The model under review builds one solid part; all positions refer to its coordinate system, in mm. A direction names the side the tool comes from. Coordinates: 2 decimals unless noted, no trailing zeros. Write each loop counter-clockwise with the first axis right and the second up, starting at its lowest first coordinate (ties: lowest second). Pieces come first, ordered by that corner, then holes. Notation, with made-up numbers: (61.5, 86.25) - (77.5, 86.25) arc R17 cw to (77.5, 114.25) - close; hole circle Ø4 at (-11, 1). An arc over 180 degrees is marked (long way). Put each result on its own line as item: value. Start each with the question number.
Item 1: Mouldability with a two-part tool opening along X and no side actions: class faces 5 (the face through (-14, 40, 0)), 6 (the face through (-17.8, 48.5, -15.9)), 7 (the face through (-23.846, 4.93, -7.509)) as pulls with the +X half, pulls with the -X half, needs draft (parallel to the pull), parting line crosses it, or undercut.
Item 2: Consider section A-A on x = 0. Give the boundary of the cut face in (y, z).
Item 3: For pin 1 (4.5 mm diameter, centred on x = 11.14, z = -11.14, fed in from -Y); pin 2 (3 mm diameter, centred on x = -21, z = 13.5, fed in from +Y); pin 3 (8 mm diameter, centred on y = 11.5, z = -3.5, fed in from +X), all flat-tipped, find the tip position at first contact; note any pin that passes through.
Item 4: Consider section D-D on y = 39. Give the boundary of the cut face in (x, z).
Item 5: To check wall thickness, follow L1, parallel to X at y = 2, z = 0; L2, parallel to X at y = 43, z = 13; L3, parallel to Y at x = -3, z = -21.5. State the ranges of each line that lie inside material, in increasing order. Write a range as [from, to].
Item 6: Machinability: for faces 1 (the face through (16, 10, 0)), 2 (the face through (-23, 47, -13)), 3 (the face through (11, 0, -17)), 4 (the face through (-10.31, 7.46, -13.76)), which of the approach directions +Z, -Z, +X, -X, +Y, -Y give a long, thin tool a straight path to every point of the face, cutting with its end or side? Answer none if there is none.
Item 7: Consider section B-B on y = 4. Give the boundary of the cut face in (x, z), then the cut area to 3 significant figures.
Item 8: Consider section C-C on y = 15. Give the boundary of the cut face in (x, z).
```python
from build123d import *

# Parameters (mm, degrees)
F3_D            = 3.3
F3_DEPTH        = 14.1
F3_TIP          = 0.9914200214
F2_R            = 4
F4_DEPTH        = 3
F5_R            = 2.75
F6_DEPTH        = 25
F6_COPIES_COUNT = 4
F8_R            = 2
F9_DEPTH        = 25


# Not quite as in the source:
# - a pattern or mirror of a feature is missing from the dataset's text; its kind, count and spacing are read off the source's solid


with BuildPart() as f1:
    # F0 (on Top) → F1 (revolve)
    with BuildSketch(Plane.XY):
        with BuildLine():
            Line((-25, 0), (-20, 0))
            Line((-20, 0), (-20, 5))
            Line((-20, 5), (0, 5))
            Line((0, 5), (0, 50))
            Line((0, 50), (-32, 50))
            Line((-32, 50), (-32, 40))
            Line((-32, 40), (-13, 40))
            ThreePointArc((-13, 40), (-10.8786796564, 39.1213203436), (-10, 37))
            Line((-10, 37), (-10, 13))
            ThreePointArc((-10, 13), (-10.8786796564, 10.8786796564), (-13, 10))
            Line((-13, 10), (-25, 10))
            Line((-25, 10), (-25, 0))
        make_face()
    revolve(axis=Axis((0, 27.5, 0), (0, -1, 0)))

    # F3
    with Locations(Plane(origin=(0, 50, 0), x_dir=(-1, 0, 0), z_dir=(0, 1, 0))):
        with Locations((21, -13.5), (21, 13.5), (-21, 13.5), (-21, -13.5)):
            Hole(F3_D / 2, depth=F3_DEPTH)
            with Locations((0, 0, -(F3_DEPTH + F3_TIP / 2))):  # 118° drill point
                Cone(0, F3_D / 2, F3_TIP, mode=Mode.SUBTRACT)

    # F2 (on face) → F4 (cut)
    with BuildSketch(Plane(origin=(0, 50, 0), x_dir=(-1, 0, 0), z_dir=(0, 1, 0))):
        with Locations((21, -13.5)):
            Circle(F2_R)
        with Locations((-21, 13.5)):
            Circle(F2_R)
    extrude(amount=-F4_DEPTH, mode=Mode.SUBTRACT)

    # F5 (on face) → F6 (cut)
    with BuildSketch(Plane.XZ.offset(-5)):
        with Locations((11.1369318037, -11.1369318037)):
            Circle(F5_R)
    f6 = extrude(amount=-F6_DEPTH, mode=Mode.SUBTRACT)

    # F6_copies: F6 ×4 about axis
    f6_copies_axis = Axis((0, 0, 0), (0, 1, 0))
    for i in range(1, F6_COPIES_COUNT):
        add(f6.rotate(f6_copies_axis, i * 360 / F6_COPIES_COUNT), mode=Mode.SUBTRACT)

    # F8 (on face) → F9 (cut)
    with BuildSketch(Plane.XZ.offset(-5)):
        with Locations((0, 15.75)):
            Circle(F8_R)
    extrude(amount=-F9_DEPTH, mode=Mode.SUBTRACT)


solid = f1.part
```
Report:
1. face 5: needs draft
1. face 6: undercut
1. face 7: parting line crosses it
2. outline: (0, -25) - (10, -25) - (10, -13) arc R3 cw to (13, -10) - (37, -10) arc R3 cw to (40, -13) - (40, -32) - (50, -32) - (50, 32) - (40, 32) - (40, 13) arc R3 cw to (37, 10) - (13, 10) arc R3 cw to (10, 13) - (10, 13.75) - (5, 13.75) - (5, -20) - (0, -20) - close; (0, 20) - (5, 20) - (5, 17.75) - (10, 17.75) - (10, 25) - (0, 25) - close
3. pin 1: y = 40
3. pin 2: y = 10
3. pin 3: x = 25
4. outline: circle Ø21.53 at (0, 0)
5. L1: [-25, -20], [20, 25]
5. L2: [-29.24, -22.57], [-19.43, 19.43], [22.57, 29.24]
5. L3: [0, 10], [40, 50]
6. face 1: none
6. face 2: +Y
6. face 3: +Z, -Z, +X, -X, -Y
6. face 4: -Y
7. outline: circle Ø50 at (0, 0); hole circle Ø40 at (0, 0)
7. area: 707 mm²
8. outline: circle Ø20 at (0, 0)
